The figure shows three views and two pictorial views of one solid part (mm, origin at its lowest corner). Answer the questions. Round coordinates to 2 decimals unless told otherwise and drop trailing zeros. Order: outer loops, then holes, each group sorted by start corner. A loop starts at its lowest first (then second) coordinate and runs counter-clockwise, first axis right, second up. Notation, with made-up numbers: (-35.5, 56.25) -> (19.5, 56.25) arc R12 ccw to (19.5, 75.25) -> close; hole circle Ø9 at (-17.5, 51). An arc over 180 degrees is marked (long way). One line per item, written item: value. Start each with the question number.
1. Section A-A (y = 4.5) is taken. Give the vertices of the cut face in (x, z).
2. Section B-B (x = 26.5) is taken. Give the vertices of the cut face in (y, z), then the cut area to 3 significant figures.
3. Flat-ended cylindrical pins translate along their axes: pin 1 Ø1.5 at (y, z) = (2.5, 2) entering from -X; pin 2 Ø3 at (y, z) = (3, 15.5) entering from +X; pin 3 Ø3 at (x, y) = (24, 4) entering from +Z. Find the tip coordinate at first contact, or state that the pin passes through.
4. Consider line 1 (X direction, y = 0.55, z = 28); line 2 (Z direction, x = 15.5, y = 0.95); line 3 (Z direction, x = 234, y = 4.95). Determine where each line is inside the solid, lowest interval first.
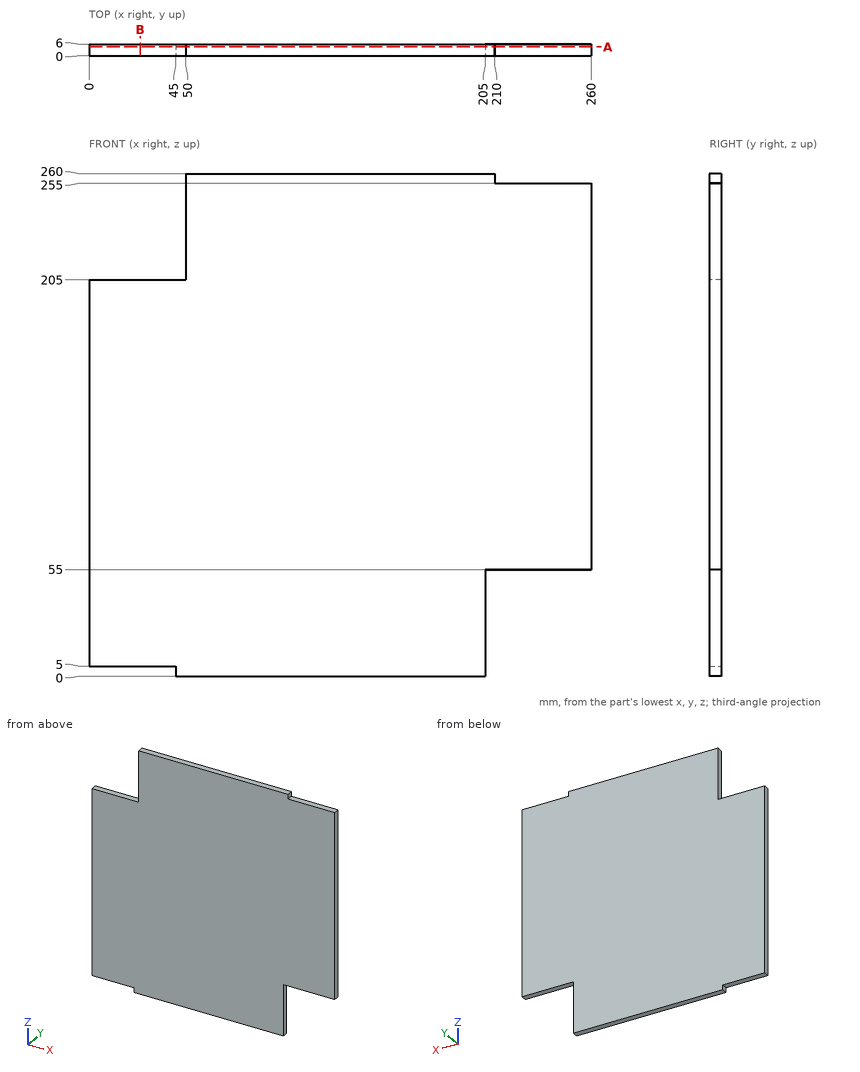
Answer:
1. outline: (0, 5) -> (45, 5) -> (45, 0) -> (205, 0) -> (205, 55) -> (260, 55) -> (260, 255) -> (210, 255) -> (210, 260) -> (50, 260) -> (50, 205) -> (0, 205) -> close
2. outline: (0, 5) -> (6, 5) -> (6, 205) -> (0, 205) -> close
2. area: 1,200 mm^2
3. pin 1: x = 45
3. pin 2: x = 205
3. pin 3: z = 205
4. line 1: 0 to 205
4. line 2: 5 to 205
4. line 3: 55 to 255
